Geometry: final body of the model. Coordinates: model frame, mm. Face numbers are marked on the shaded views. Round coordinates to 2 decimals unless told otherwise and drop trailing zeros. Write each loop counter-clockwise with the first axis right and the second up, starting at its lowest first coordinate (ties: lowest second). Pieces come first, ordered by that corner, then holes. Notation, with made-up numbers: M 86,-40 L 136,-40 A25 cw 136,-14 Z; hole C 31.25,40.5 d8. An arc over 180 degrees is marked long. Use one line per item in the form item = value. Start each with the question number.
Item 1: Section query C-C (y = 3.4). Return loops of the section in (x, z), and give its area (3 significant figures).
Item 2: Section query D-D (x = -221). Return loops of the section in (y, z), and give its area (3 significant figures).
Item 3: Ray query, probe 1 along X at (y, z) = (1.5, -121); probe 2 along Z at (x, y) = (-198, 0.3); probe 3 along X at (y, z) = (0.9, -106). Return the intervals inside material, ascending.
Item 4: Pin query (flat end, axial travel): pin 1 Ø4.5 at (x, z) = (-184.84, -36.12) entering from -Y; pin 2 Ø1.5 at (x, z) = (-216, -105) entering from +Y; pin 3 Ø2.5 at (x, z) = (-215, -37.5) entering from +Y. Return the tip coordinate at first contact, or that it passes through.
Item 5: Section query B-B (z = -78). Return loops of the section in (x, y), and give its area (3 significant figures).
Item 6: Section query A-A (x = -204.5). Return loops of the section in (y, z).
Item 7: Pull-direction query (Z, two-part tool) for the marked faces 1 and 2; classes: pulls with the +Z half, pulls with the -Z half, needs draft (parallel to the pull), parting line crosses it, or undercut.
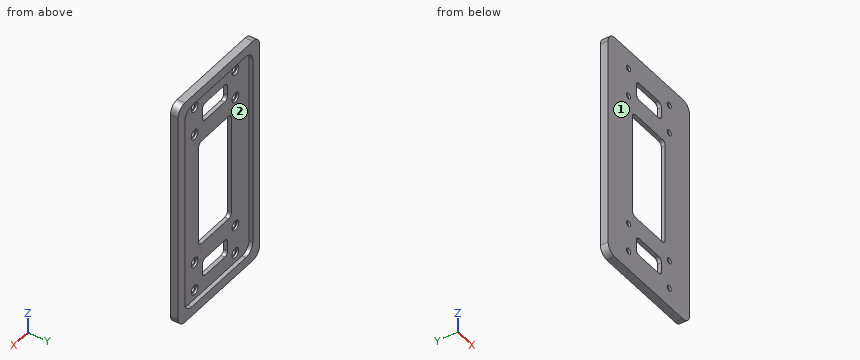
from build123d import *

# Parameters (mm, degrees)
EXTRUDE_1_DEPTH = 4
SKETCH_1_40_R   = 2.5
EXTRUDE_2_DEPTH = 2
SKETCH_1_41_R   = 2.5
SKETCH_1_41_R_2 = 1.5
EXTRUDE_3_DEPTH = 1


with BuildPart() as part:
    # Sketch 1 → Extrude 1 (new body)
    with BuildSketch(Plane(origin=(0, 0, 0), x_dir=(1, 0, 0), z_dir=(0, 1, 0))):
        with BuildLine():
            ThreePointArc((-169.840079727, 16.119726246), (-171.304545821, 12.58419234), (-174.840079727, 11.119726246))
            Line((-174.840079727, 11.119726246), (-199.840079727, 11.119726246))
            Line((-199.840079727, 11.119726246), (-224.840079727, 11.119726246))
            ThreePointArc((-224.840079727, 11.119726246), (-228.375613633, 12.58419234), (-229.840079727, 16.119726246))
            Line((-229.840079727, 16.119726246), (-229.840079727, 126.119726246))
            ThreePointArc((-229.840079727, 126.119726246), (-228.375613633, 129.655260152), (-224.840079727, 131.119726246))
            Line((-224.840079727, 131.119726246), (-199.840079727, 131.119726246))
            Line((-199.840079727, 131.119726246), (-174.840079727, 131.119726246))
            ThreePointArc((-174.840079727, 131.119726246), (-171.304545821, 129.655260152), (-169.840079727, 126.119726246))
            Line((-169.840079727, 126.119726246), (-169.840079727, 16.119726246))
        make_face()
        with BuildLine():
            Line((-224.840079727, 21.119726246), (-224.840079727, 121.119726246))
            ThreePointArc((-224.840079727, 121.119726246), (-223.375613633, 124.655260152), (-219.840079727, 126.119726246))
            Line((-219.840079727, 126.119726246), (-179.840079727, 126.119726246))
            ThreePointArc((-179.840079727, 126.119726246), (-176.304545821, 124.655260152), (-174.840079727, 121.119726246))
            Line((-174.840079727, 121.119726246), (-174.840079727, 21.119726246))
            ThreePointArc((-174.840079727, 21.119726246), (-176.304545821, 17.58419234), (-179.840079727, 16.119726246))
            Line((-179.840079727, 16.119726246), (-219.840079727, 16.119726246))
            ThreePointArc((-219.840079727, 16.119726246), (-223.375613633, 17.58419234), (-224.840079727, 21.119726246))
        make_face(mode=Mode.SUBTRACT)
    extrude(amount=EXTRUDE_1_DEPTH)

    # Sketch 1_40 → Extrude 2 (add)
    with BuildSketch(Plane(origin=(0, 0, 0), x_dir=(1, 0, 0), z_dir=(0, 1, 0))):
        with BuildLine():
            ThreePointArc((-224.840079727, 121.119726246), (-223.375613633, 124.655260152), (-219.840079727, 126.119726246))
            Line((-219.840079727, 126.119726246), (-179.840079727, 126.119726246))
            ThreePointArc((-179.840079727, 126.119726246), (-176.304545821, 124.655260152), (-174.840079727, 121.119726246))
            Line((-174.840079727, 121.119726246), (-174.840079727, 21.119726246))
            ThreePointArc((-174.840079727, 21.119726246), (-176.304545821, 17.58419234), (-179.840079727, 16.119726246))
            Line((-179.840079727, 16.119726246), (-219.840079727, 16.119726246))
            ThreePointArc((-219.840079727, 16.119726246), (-223.375613633, 17.58419234), (-224.840079727, 21.119726246))
            Line((-224.840079727, 21.119726246), (-224.840079727, 121.119726246))
        make_face()
        with Locations(Location((-184.840079727, 36.119726246, 0), (0, 0, 270))):
            Circle(SKETCH_1_40_R, mode=Mode.SUBTRACT)
        with Locations(Location((-214.840082087, 106.119726246, 0), (0, 0, 270))):
            Circle(SKETCH_1_40_R, mode=Mode.SUBTRACT)
        with Locations(Location((-214.840082087, 21.119726246, 0), (0, 0, 270))):
            Circle(SKETCH_1_40_R, mode=Mode.SUBTRACT)
        with Locations(Location((-214.840082087, 121.119726246, 0), (0, 0, 270))):
            Circle(SKETCH_1_40_R, mode=Mode.SUBTRACT)
        with Locations(Location((-184.840079727, 121.119726246, 0), (0, 0, 270))):
            Circle(SKETCH_1_40_R, mode=Mode.SUBTRACT)
        with Locations(Location((-184.840079727, 21.119726246, 0), (0, 0, 270))):
            Circle(SKETCH_1_40_R, mode=Mode.SUBTRACT)
        with Locations(Location((-214.840082087, 36.119726246, 0), (0, 0, 270))):
            Circle(SKETCH_1_40_R, mode=Mode.SUBTRACT)
        with Locations(Location((-184.840079727, 106.119726246, 0), (0, 0, 270))):
            Circle(SKETCH_1_40_R, mode=Mode.SUBTRACT)
        with BuildLine():
            ThreePointArc((-209.782711851, 99.187170628), (-211.257930865, 98.576114904), (-211.868986589, 97.10089589))
            Line((-211.868986589, 97.10089589), (-211.868986589, 45.138556602))
            ThreePointArc((-211.868986589, 45.138556602), (-211.257930865, 43.663337587), (-209.782711851, 43.052281864))
            Line((-209.782711851, 43.052281864), (-189.897449963, 43.052281864))
            ThreePointArc((-189.897449963, 43.052281864), (-188.422230949, 43.663337587), (-187.811175226, 45.138556602))
            Line((-187.811175226, 45.138556602), (-187.811175226, 97.10089589))
            ThreePointArc((-187.811175226, 97.10089589), (-188.422230949, 98.576114904), (-189.897449963, 99.187170628))
            Line((-189.897449963, 99.187170628), (-209.782711851, 99.187170628))
        make_face(mode=Mode.SUBTRACT)
        with BuildLine():
            Line((-209.073480954, 31.150151169), (-209.073480954, 26.089301323))
            ThreePointArc((-209.073480954, 26.089301323), (-208.462425231, 24.614082309), (-206.987206217, 24.003026586))
            Line((-206.987206217, 24.003026586), (-192.692955598, 24.003026586))
            ThreePointArc((-192.692955598, 24.003026586), (-191.217736584, 24.614082309), (-190.606680861, 26.089301323))
            Line((-190.606680861, 26.089301323), (-190.606680861, 31.150151169))
            ThreePointArc((-190.606680861, 31.150151169), (-191.217736584, 32.625370183), (-192.692955598, 33.236425906))
            Line((-192.692955598, 33.236425906), (-206.987206217, 33.236425906))
            ThreePointArc((-206.987206217, 33.236425906), (-208.462425231, 32.625370183), (-209.073480954, 31.150151169))
        make_face(mode=Mode.SUBTRACT)
        with BuildLine():
            Line((-209.073480954, 111.089301323), (-209.073480954, 116.150151169))
            ThreePointArc((-209.073480954, 116.150151169), (-208.462425231, 117.625370183), (-206.987206217, 118.236425906))
            Line((-206.987206217, 118.236425906), (-192.692955598, 118.236425906))
            ThreePointArc((-192.692955598, 118.236425906), (-191.217736584, 117.625370183), (-190.606680861, 116.150151169))
            Line((-190.606680861, 116.150151169), (-190.606680861, 111.089301323))
            ThreePointArc((-190.606680861, 111.089301323), (-191.217736584, 109.614082309), (-192.692955598, 109.003026586))
            Line((-192.692955598, 109.003026586), (-206.987206217, 109.003026586))
            ThreePointArc((-206.987206217, 109.003026586), (-208.462425231, 109.614082309), (-209.073480954, 111.089301323))
        make_face(mode=Mode.SUBTRACT)
    extrude(amount=EXTRUDE_2_DEPTH)

    # Sketch 1_41 → Extrude 3 (add)
    # profile 1 of 8: a face of its own
    with BuildSketch(Plane(origin=(0, 0, 0), x_dir=(1, 0, 0), z_dir=(0, 1, 0))):
        with Locations(Location((-214.840082087, 36.119726246, 0), (0, 0, 270))):
            Circle(SKETCH_1_41_R)
        with Locations(Location((-214.840082087, 36.119726246, 0), (0, 0, 270))):
            Circle(SKETCH_1_41_R_2, mode=Mode.SUBTRACT)
    # profile 2 of 8: a face of its own
    with BuildSketch(Plane(origin=(0, 0, 0), x_dir=(1, 0, 0), z_dir=(0, 1, 0))):
        with Locations(Location((-214.840082087, 21.119726246, 0), (0, 0, 270))):
            Circle(SKETCH_1_41_R)
        with Locations(Location((-214.840082087, 21.119726246, 0), (0, 0, 270))):
            Circle(SKETCH_1_41_R_2, mode=Mode.SUBTRACT)
    # profile 3 of 8: a face of its own
    with BuildSketch(Plane(origin=(0, 0, 0), x_dir=(1, 0, 0), z_dir=(0, 1, 0))):
        with Locations(Location((-184.840079727, 21.119726246, 0), (0, 0, 270))):
            Circle(SKETCH_1_41_R)
        with Locations(Location((-184.840079727, 21.119726246, 0), (0, 0, 270))):
            Circle(SKETCH_1_41_R_2, mode=Mode.SUBTRACT)
    # profile 4 of 8: a face of its own
    with BuildSketch(Plane(origin=(0, 0, 0), x_dir=(1, 0, 0), z_dir=(0, 1, 0))):
        with Locations(Location((-184.840079727, 36.119726246, 0), (0, 0, 270))):
            Circle(SKETCH_1_41_R)
        with Locations(Location((-184.840079727, 36.119726246, 0), (0, 0, 270))):
            Circle(SKETCH_1_41_R_2, mode=Mode.SUBTRACT)
    # profile 5 of 8: a face of its own
    with BuildSketch(Plane(origin=(0, 0, 0), x_dir=(1, 0, 0), z_dir=(0, 1, 0))):
        with Locations(Location((-214.840082087, 106.119726246, 0), (0, 0, 270))):
            Circle(SKETCH_1_41_R)
        with Locations(Location((-214.840082087, 106.119726246, 0), (0, 0, 270))):
            Circle(SKETCH_1_41_R_2, mode=Mode.SUBTRACT)
    # profile 6 of 8: a face of its own
    with BuildSketch(Plane(origin=(0, 0, 0), x_dir=(1, 0, 0), z_dir=(0, 1, 0))):
        with Locations(Location((-214.840082087, 121.119726246, 0), (0, 0, 270))):
            Circle(SKETCH_1_41_R)
        with Locations(Location((-214.840082087, 121.119726246, 0), (0, 0, 270))):
            Circle(SKETCH_1_41_R_2, mode=Mode.SUBTRACT)
    # profile 7 of 8: a face of its own
    with BuildSketch(Plane(origin=(0, 0, 0), x_dir=(1, 0, 0), z_dir=(0, 1, 0))):
        with Locations(Location((-184.840079727, 121.119726246, 0), (0, 0, 270))):
            Circle(SKETCH_1_41_R)
        with Locations(Location((-184.840079727, 121.119726246, 0), (0, 0, 270))):
            Circle(SKETCH_1_41_R_2, mode=Mode.SUBTRACT)
    # profile 8 of 8: a face of its own
    with BuildSketch(Plane(origin=(0, 0, 0), x_dir=(1, 0, 0), z_dir=(0, 1, 0))):
        with Locations(Location((-184.840079727, 106.119726246, 0), (0, 0, 270))):
            Circle(SKETCH_1_41_R)
        with Locations(Location((-184.840079727, 106.119726246, 0), (0, 0, 270))):
            Circle(SKETCH_1_41_R_2, mode=Mode.SUBTRACT)
    extrude(amount=EXTRUDE_3_DEPTH)


solid = part.part
Working result:
q1.outline = M -229.84,-126.12 A5 ccw -224.84,-131.12 L -174.84,-131.12 A5 ccw -169.84,-126.12 L -169.84,-16.12 A5 ccw -174.84,-11.12 L -224.84,-11.12 A5 ccw -229.84,-16.12 Z; hole M -224.84,-121.12 A5 ccw -219.84,-126.12 L -179.84,-126.12 A5 ccw -174.84,-121.12 L -174.84,-21.12 A5 ccw -179.84,-16.12 L -219.84,-16.12 A5 ccw -224.84,-21.12 Z
q1.area = 1,700 mm²
q2.outline = M 0,-131.12 L 4,-131.12 L 4,-125.98 L 2,-125.98 L 2,-16.26 L 4,-16.26 L 4,-11.12 L 0,-11.12 Z
q2.area = 261 mm²
q3.probe_1 = -229.84 to -217.34, -212.34 to -187.34, -182.34 to -169.84
q3.probe_2 = -131.12 to -118.24, -109 to -99.19, -43.05 to -33.24, -24 to -11.12
q3.probe_3 = -229.84 to -216.34, -213.34 to -186.34, -183.34 to -169.84
q4.pin_1 = 0
q4.pin_2 = 1
q4.pin_3 = 2
q5.outline = M -229.84,0 L -211.87,0 L -211.87,2 L -224.84,2 L -224.84,4 L -229.84,4 Z; M -187.81,0 L -169.84,0 L -169.84,4 L -174.84,4 L -174.84,2 L -187.81,2 Z
q5.area = 91.9 mm²
q6.outline = M 0,-131.12 L 4,-131.12 L 4,-126.12 L 2,-126.12 L 2,-118.24 L 0,-118.24 Z; M 0,-109 L 2,-109 L 2,-99.19 L 0,-99.19 Z; M 0,-43.05 L 2,-43.05 L 2,-33.24 L 0,-33.24 Z; M 0,-24 L 2,-24 L 2,-16.12 L 4,-16.12 L 4,-11.12 L 0,-11.12 Z
q7.face_1 = needs draft
q7.face_2 = undercut
